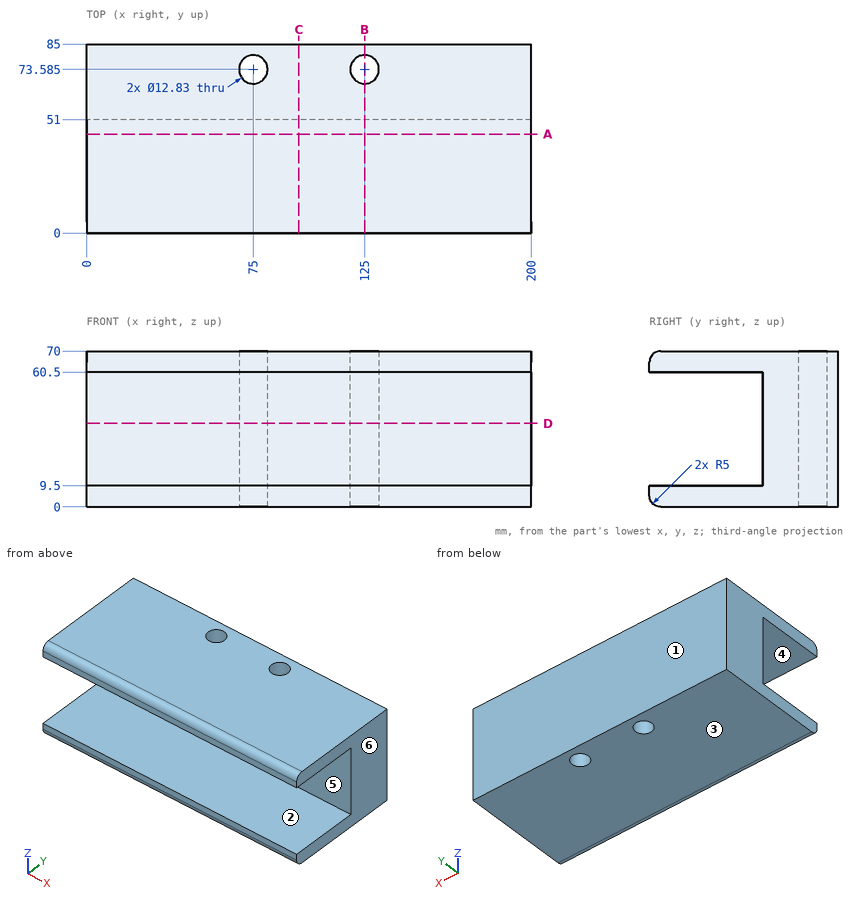
Input: dimensioned drawing with shaded views. Units: mm. Origin: part minimum x, y, z. A direction names the side the tool comes from. Round coordinates to 2 decimals unless told otherwise and drop trailing zeros. Loops run counter-clockwise (first coordinate to the right, second up) from the corner with the lowest first, then second, coordinate; pieces in that order, holes last. Notation, with made-up numbers: M 40,21 L 63,21 A22 cw 63,34 Z; hole C -11,79 d10. An arc over 180 degrees is marked long. Return JSON: item names as keys, results as strings. Group by question number.
1. Reachability of the marked faces 1 and 2 from +Z, -Z, +X, -X, +Y, -Y: full face, straight path, thin tool, end or side. Return the list, or none.
2. Section query D-D on z = 37.5. Output: boundary loops of the cut face in (x, y) (3 decimals), and give its area (3 significant figures).
3. Mould query, pull axis Z, two halves, no side actions, for the marked faces 3, 4, 5 and 6. Classes: released by +Z, released by -Z, zero draft, split by the parting line, or undercut.
4. Pin query (flat end, axial travel): pin 1 (4 mm diameter, centred on x = 34, z = 23, fed in from -Y). Return the tip coordinate at first contact, or that it passes through.
5. Section query C-C on x = 95.5. Output: boundary loops of the cut face in (y, z).
6. Section query A-A on y = 44.5. Output: boundary loops of the cut face in (x, z).
7. Section query B-B on x = 125. Output: boundary loops of the cut face in (y, z), and give its area (3 significant figures).
8. Material intervals for line 1 along Z through (x, y) = (60, 24); line 2 along X through (y, z) = (73.5, 49); line 3 along Y through (x, z) = (125, 20), sorted ascending. Write a range as from..to.
Checks:
{
 "1": {"face 1": "+Z, -Z, +X, -X, +Y", "face 2": "+X, -X, -Y"},
 "2": {"outline": "M 0,51 L 200,51 L 200,85 L 0,85 Z; hole C 75,73.585 d12.83; hole C 125,73.585 d12.83", "area": "6,540 mm²"},
 "3": {"face 3": "released by -Z", "face 4": "undercut", "face 5": "undercut", "face 6": "zero draft"},
 "4": {"pin 1": "stops at y = 51"},
 "5": {"outline": "M 0,5 A5 ccw 5,0 L 85,0 L 85,70 L 5,70 A5 ccw 0,65 L 0,60.5 L 51,60.5 L 51,9.5 L 0,9.5 Z"},
 "6": {"outline": "M 0,0 L 200,0 L 200,9.5 L 0,9.5 Z; M 0,60.5 L 200,60.5 L 200,70 L 0,70 Z"},
 "7": {"outline": "M 0,5 A5 ccw 5,0 L 67.17,0 L 67.17,70 L 5,70 A5 ccw 0,65 L 0,60.5 L 51,60.5 L 51,9.5 L 0,9.5 Z; M 80,0 L 85,0 L 85,70 L 80,70 Z", "area": "2,440 mm²"},
 "8": {"line 1": "z = 0..9.5, 60.5..70", "line 2": "x = 0..68.59, 81.41..118.59, 131.41..200", "line 3": "y = 51..67.17, 80..85"}
}
